Check sheet for the modelled part. Datum: model origin and axes. Units: mm. Give positions to 0.01 mm unless a question says otherwise; leave off trailing zeros. Order: outer loops, then holes, each group sorted by start corner. A loop starts at its lowest first (then second) coordinate and runs counter-clockwise, first axis right, second up.
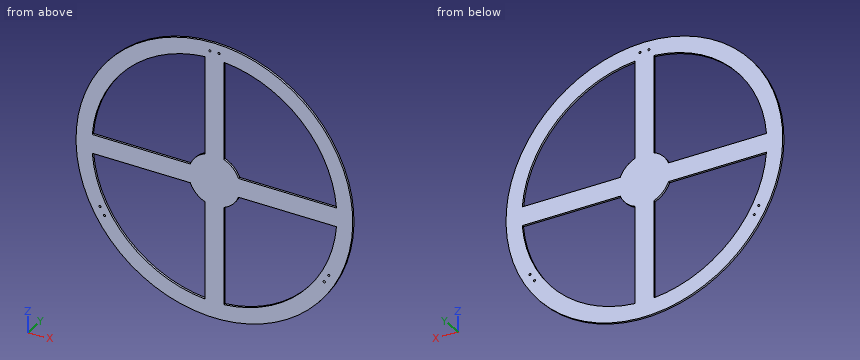
```python
from build123d import *

# Parameters (mm, degrees)
SKETCH1_R           = 196.85
SKETCH1_R_2         = 1.5
BOSS_EXTRUDE1_DEPTH = 3


with BuildPart() as part:
    # Sketch1 → Boss-Extrude1 (new body)
    with BuildSketch(Plane(origin=(0, 0, 0), x_dir=(1, 0, 0), z_dir=(0, 1, 0))):
        with Locations(Location((479.721156758, 531.943650225, 0), (0, 0, 270))):
            Circle(SKETCH1_R)
        with Locations(Location((473.371156758, 347.793650225, 0), (0, 0, 270))):
            Circle(SKETCH1_R_2, mode=Mode.SUBTRACT)
        with Locations(Location((486.071156758, 347.793650225, 0), (0, 0, 270))):
            Circle(SKETCH1_R_2, mode=Mode.SUBTRACT)
        with Locations(Location((323.417578651, 629.517911539, 0), (0, 0, 270))):
            Circle(SKETCH1_R_2, mode=Mode.SUBTRACT)
        with Locations(Location((317.067578651, 618.519388911, 0), (0, 0, 270))):
            Circle(SKETCH1_R_2, mode=Mode.SUBTRACT)
        with Locations(Location((642.374734865, 618.519388911, 0), (0, 0, 270))):
            Circle(SKETCH1_R_2, mode=Mode.SUBTRACT)
        with Locations(Location((636.024734865, 629.517911539, 0), (0, 0, 270))):
            Circle(SKETCH1_R_2, mode=Mode.SUBTRACT)
        with BuildLine():
            Line((653.442357833, 518.540768582), (514.055823837, 518.540768582))
            ThreePointArc((514.055823837, 518.540768582), (505.783645125, 505.881161858), (493.124038401, 497.608983146))
            Line((493.124038401, 497.608983146), (493.124038401, 358.22244915))
            ThreePointArc((493.124038401, 358.22244915), (602.925647219, 408.739159764), (653.442357833, 518.540768582))
        make_face(mode=Mode.SUBTRACT)
        with BuildLine():
            Line((305.999955683, 518.540768582), (445.386489679, 518.540768582))
            ThreePointArc((445.386489679, 518.540768582), (453.658668391, 505.881161858), (466.318275115, 497.608983146))
            Line((466.318275115, 497.608983146), (466.318275115, 358.22244915))
            ThreePointArc((466.318275115, 358.22244915), (356.516666298, 408.739159764), (305.999955683, 518.540768582))
        make_face(mode=Mode.SUBTRACT)
        with BuildLine():
            Line((653.442357833, 545.346531867), (514.055823837, 545.346531867))
            ThreePointArc((514.055823837, 545.346531867), (505.783645125, 558.006138591), (493.124038401, 566.278317303))
            Line((493.124038401, 566.278317303), (493.124038401, 705.6648513))
            ThreePointArc((493.124038401, 705.6648513), (602.925647219, 655.148140685), (653.442357833, 545.346531867))
        make_face(mode=Mode.SUBTRACT)
        with BuildLine():
            Line((445.386489679, 545.346531867), (305.999955683, 545.346531867))
            ThreePointArc((305.999955683, 545.346531867), (356.516666298, 655.148140685), (466.318275115, 705.6648513))
            Line((466.318275115, 705.6648513), (466.318275115, 566.278317303))
            ThreePointArc((466.318275115, 566.278317303), (453.658668391, 558.006138591), (445.386489679, 545.346531867))
        make_face(mode=Mode.SUBTRACT)
    extrude(amount=BOSS_EXTRUDE1_DEPTH)


solid = part.part
```
(1) Sectioned sample at B-B (z = -401.5). Enter the section's corners in (x, y), plus the area to 3 significant figures.
(2) Sectioned sample at A-A (x = 424). Enter the section's corners in (y, z), plus the area to 3 significant figures.
(3) Thickness scan on L1, parallel to X at y = 0.35, z = -551; L2, parallel to Z at x = 502, y = 1.5; L3, parallel to Z at x = 460, y = 1.75. Record the ranges inside material, lowest first.
(4) Go/stop test with flat-tipped pins: P1, Ø1.5, axis at y = 2, z = -393.5, coming from the +X side; P2, Ø0.9, axis at y = 1.5, z = -462, coming from the -X side; P3, Ø1.5, axis at y = 1, z = -628, coming from the +X side. Record where each tip stops, or that it passes through.
(5) Sectioned sample at C-C (y = 1.9). Count the separate pieces of the cut face and the enclosed holes in it, plus the area to 3 significant figures.
Values follow:
1. outline: (332.3, 0) - (364.21, 0) - (364.21, 3) - (332.3, 3) - close; (466.32, 0) - (493.12, 0) - (493.12, 3) - (466.32, 3) - close; (595.23, 0) - (627.15, 0) - (627.15, 3) - (595.23, 3) - close
1. area: 272 mm2
2. outline: (0, -720.74) - (3, -720.74) - (3, -697.03) - (0, -697.03) - close; (0, -545.35) - (3, -545.35) - (3, -518.54) - (0, -518.54) - close; (0, -366.86) - (3, -366.86) - (3, -343.14) - (0, -343.14) - close
2. area: 223 mm2
3. L1: x = 283.8 to 306.53, 448.17 to 511.27, 652.91 to 675.65
3. L2: z = -727.53 to -704.75, -561.31 to -502.58, -359.14 to -336.36
3. L3: z = -727.8 to -705.06, -563.08 to -500.81, -358.83 to -336.08
4. P1: stops at x = 620.4
4. P2: stops at x = 295.55
4. P3: stops at x = 651.96
5. separate pieces: 1
5. enclosed holes: 10
5. area: 45,400 mm2
